The drawing under review shows one solid part. Ordinate dimensions are in mm from its lowest x, y, z. Coordinates: 2 decimals unless noted, no trailing zeros. Write each loop counter-clockwise with the first axis right and the second up, starting at its lowest first coordinate (ties: lowest second). Pieces come first, ordered by that corner, then holes. Notation, with made-up numbers: (66, 62.25) - (73, 62.25) arc R23 cw to (73, 97.25) - close; hole circle Ø5 at (-20.5, 81.25). An arc over 180 degrees is marked (long way). Use a Markdown table: item, result.
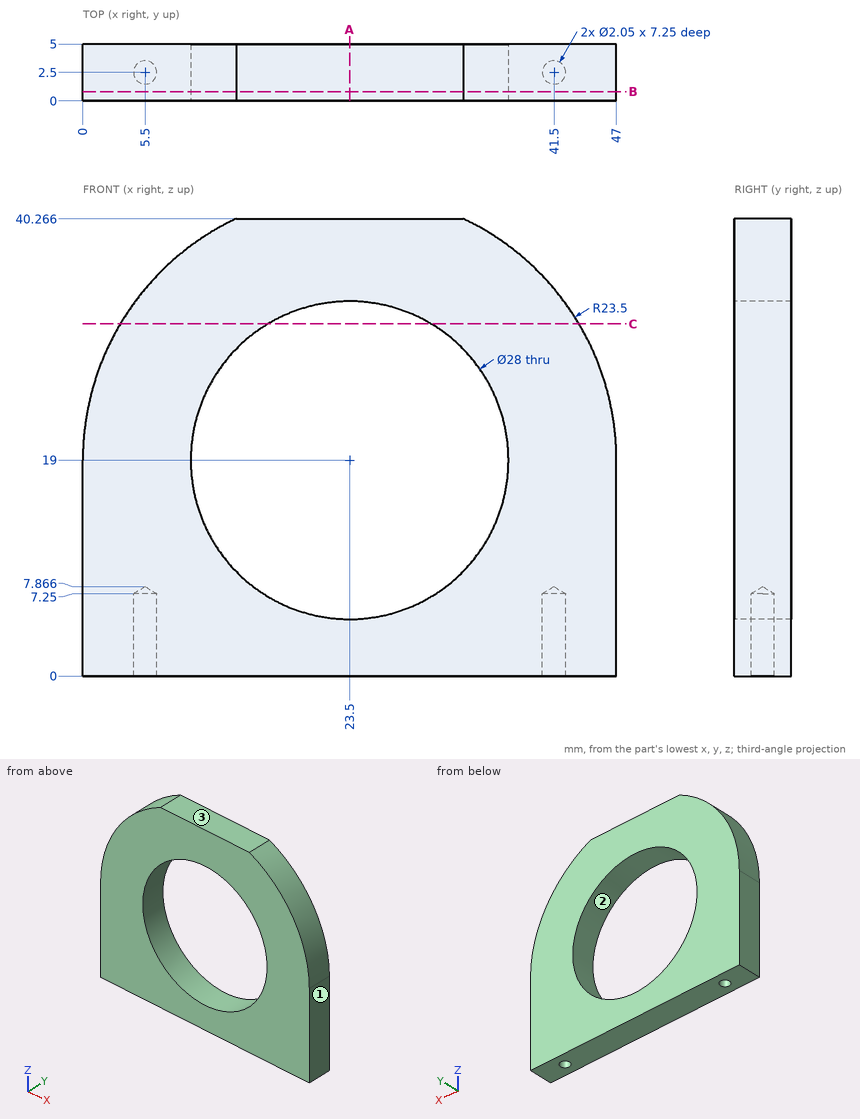
(1) Draft analysis for pull direction Z (two halves, no side actions). For the marked faces 1, 2 and 3, state which applies: +Z half, -Z half, draft (parallel to the pull), parting line (faces both ways), or undercut.
Determined:
| item | result |
|---|---|
| face 1 | draft |
| face 2 | undercut |
| face 3 | +Z half |
(2) Take a section at C-C on z = 31. Write out the cut boundary in (x, y) (1 decimal).
Determined:
| item | result |
|---|---|
| outline | (3.3, 0) - (16.3, 0) - (16.3, 5) - (3.3, 5) - close; (30.7, 0) - (43.7, 0) - (43.7, 5) - (30.7, 5) - close |
(3) For L1, parallel to X at y = 2.5, z = 3.75 (3 decimals); L2, parallel to Y at x = 5.5, z = 5.75 (3 decimals); L3, parallel to Z at x = 9, y = 1.35, list the stretches that pass through material, from the lowest coordinate up. Write a range as from..to.
Determined:
| item | result |
|---|---|
| L1 | 0..4.475, 6.525..40.475, 42.525..47 |
| L2 | 0..1.475, 3.525..5 |
| L3 | 0..37.49 |
(4) For pin 1 (2 mm diameter, centred on y = 1, z = 34.5, fed in from +X); pin 2 (1.6 mm diameter, centred on x = 5.5, y = 2.5, fed in from +Z); pin 3 (1 mm diameter, centred on y = 4, z = 22, fed in from -X), all flat-tipped, find the tip position at first contact; note any pin that passes through.
Determined:
| item | result |
|---|---|
| pin 1 | x = 41.99 |
| pin 2 | z = 35.01 |
| pin 3 | x = 0.13 |
(5) Take a section at B-B on y = 0.8. Write out the cut boundary in (x, z).
Determined:
| item | result |
|---|---|
| outline | (0, 0) - (47, 0) - (47, 19) arc R23.5 ccw to (33.5, 40.27) - (13.5, 40.27) arc R23.5 ccw to (0, 19) - close; hole circle Ø28 at (23.5, 19) |
(6) Take a section at A-A on x = 23.5. Write out the cut boundary in (y, z), and give its area (3 significant figures).
Determined:
| item | result |
|---|---|
| outline | (0, 0) - (5, 0) - (5, 5) - (0, 5) - close; (0, 33) - (5, 33) - (5, 40.27) - (0, 40.27) - close |
| area | 61.3 mm2 |
